```python
from build123d import *

# Parameters (mm, degrees)
SKETCH_R        = 6.5
SKETCH_R_2      = 3
SKETCH_R_3      = 20
PAD014_DEPTH    = 8
SKETCH029_R     = 10
POCKET004_DEPTH = 5
POCKET008_DEPTH = 4


with BuildPart() as part:
    # Sketch → Pad014 (new body)
    with BuildSketch(Plane.XY.offset(32)):
        Polygon((40, 192), (392, 192), (392, -182), (382, -182), (382, -192), (40, -192), align=None)
        with Locations((246.8, 50.5)):
            Circle(SKETCH_R, mode=Mode.SUBTRACT)
        with Locations((239.8, 35)):
            Circle(SKETCH_R_2, mode=Mode.SUBTRACT)
        with Locations((226.376606, 58.25)):
            Circle(SKETCH_R_2, mode=Mode.SUBTRACT)
        with Locations((253.223394, 58.25)):
            Circle(SKETCH_R_2, mode=Mode.SUBTRACT)
        with Locations((70, 180)):
            Circle(SKETCH_R_2, mode=Mode.SUBTRACT)
        with Locations((330, 180)):
            Circle(SKETCH_R_2, mode=Mode.SUBTRACT)
        with Locations((70, -180)):
            Circle(SKETCH_R_2, mode=Mode.SUBTRACT)
        with Locations((330, -180)):
            Circle(SKETCH_R_2, mode=Mode.SUBTRACT)
        with Locations((352, 140)):
            Circle(SKETCH_R_3, mode=Mode.SUBTRACT)
    extrude(amount=-PAD014_DEPTH)

    # Sketch029 → Pocket004 (cut)
    with BuildSketch(Plane.XY.offset(32)):
        with Locations((70, 180)):
            Circle(SKETCH029_R)
        with Locations((330, 180)):
            Circle(SKETCH029_R)
        with Locations((330, -180)):
            Circle(SKETCH029_R)
        with Locations((70, -180)):
            Circle(SKETCH029_R)
    extrude(amount=-POCKET004_DEPTH, mode=Mode.SUBTRACT)

    # Sketch037 → Pocket008 (cut)
    with BuildSketch(Plane(origin=(0, 0, 24), x_dir=(1, 0, 0), z_dir=(0, 0, -1))):
        with BuildLine():
            ThreePointArc((230.340527, -92.165245), (221.832227, -137.151247), (229.197543, -182.338454))
            Line((371.961304, -159.605377), (229.197543, -182.338454))
            Line((385.298035, -14.416777), (371.961304, -159.605377))
            ThreePointArc((385.298035, -14.416777), (330.776181, -12.233466), (280.15249, -32.596211))
            ThreePointArc((280.15249, -32.596211), (224.259659, -36.469349), (230.340527, -92.165245))
        make_face()
    extrude(amount=-POCKET008_DEPTH, mode=Mode.SUBTRACT)


solid = part.part
```
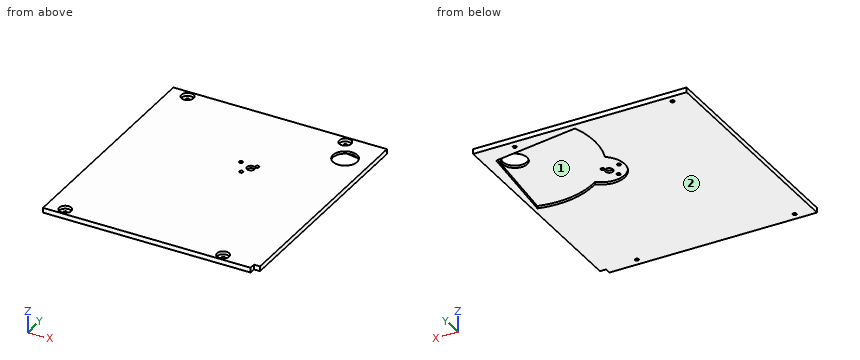
Build history of the part. All positions in model axes, mm. Face numbers are marked on the shaded views. Give positions to 0.01 mm unless a question says otherwise; leave off trailing zeros. Loops run counter-clockwise (first coordinate to the right, second up) from the corner with the lowest first, then second, coordinate; pieces in that order, holes last.
Item 1: Slice it at C-C, the plane x = 352. List the corners of the cut face in (y, z), and give its area (3 significant figures).
Answers follow:
outline: (-192, 24) - (10.33, 24) - (10.33, 28) - (120, 28) - (120, 32) - (-192, 32) - close; (160, 28) - (162.78, 28) - (162.78, 24) - (192, 24) - (192, 32) - (160, 32) - close
area: 2,300 mm2
Item 2: Flat gauge pins, fed straight in: pin 1 (9.5 mm diameter, centred on x = 70, y = 180, fed in from +Z); pin 2 (9.5 mm diameter, centred on x = 239.8, y = 35, fed in from -Z); pin 3 (2.5 mm diameter, centred on x = 386, z = 29.5, fed in from -Y). Where does each tip first touch, or does it go through?
Answers follow:
pin 1: stops at z = 27
pin 2: stops at z = 28
pin 3: stops at y = -182
Item 3: Slice it at A-A, the plane z = 25.5. List the corners of the cut face in (x, y).
Answers follow:
outline: (40, -192) - (382, -192) - (382, -182) - (392, -182) - (392, 192) - (40, 192) - close; hole circle Ø6 at (70, -180); hole circle Ø6 at (70, 180); hole (229.2, 182.34) arc R132.04 ccw to (230.34, 92.17) arc R38.86 ccw (long way) to (280.15, 32.6) arc R130.13 ccw to (385.3, 14.42) - (371.96, 159.61) - close; hole circle Ø6 at (330, -180); hole circle Ø6 at (330, 180)
Item 4: Slice it at D-D, the plane y = 97.5. List the corners of the cut face in (x, z).
Answers follow:
outline: (40, 24) - (228.45, 24) - (228.45, 28) - (377.67, 28) - (377.67, 24) - (392, 24) - (392, 32) - (40, 32) - close
Item 5: Slice it at B-B, the plane y = 140. List the corners of the cut face in (x, z).
Answers follow:
outline: (40, 24) - (221.83, 24) - (221.83, 28) - (332, 28) - (332, 32) - (40, 32) - close; (372, 28) - (373.76, 28) - (373.76, 24) - (392, 24) - (392, 32) - (372, 32) - close
Item 6: Drill centre lines: line 1 (Y direction, x = 70, z = 28.4); line 2 (Y direction, x = 246.8, z = 29.1); line 3 (Y direction, x = 72, z = 29.25). Where is each one in solid material? Low to high.
Answers follow:
line 1: y = -192 to -190, -170 to 170, 190 to 192
line 2: y = -192 to 44, 57 to 192
line 3: y = -192 to -189.8, -170.2 to 170.2, 189.8 to 192
Item 7: Pull direction X, two halves, no side cores. Call the marked faces 1 and 2: released by +X, released by -X, zero draft, split by the parting line, or undercut.
Answers follow:
face 1: undercut
face 2: zero draft
